Read the model definition and answer for the solid it produces. Units are mm, in the model's axes. A direction names the side the tool comes from. Coordinates: 2 decimals unless noted, no trailing zeros. Loops run counter-clockwise (first coordinate to the right, second up) from the corner with the lowest first, then second, coordinate; pieces in that order, holes last.
Q1. Straight lines are drawn through the part: line 1 (Y direction, x = 22.5, z = 268); line 2 (X direction, y = 24.6, z = 57.15). For each, find the intervals that lie inside material, in ascending order.
Q2. Which of the six approach directions +Z, -Z, +X, -X, +Y, -Y give full straight-line access (tool end or side, diameter ignored) to faces 4 (the face through (13, 0, 244)), 5 (the face through (23.812, 13, 243))?
Q3. The mould has two halves that part along Y. Classify faces 1 (the face through (13, 1.588, 243)), 2 (the face through (1, 13, 0)), 3 (the face through (13, 25.4, 244)): pulls with the +Y half, pulls with the -Y half, needs draft (parallel to the pull), parting line crosses it, or undercut.
Q4. Section A-A (z = 274) is taken. Give the vertices of the cut face in (x, y).
Autodesk Inventor part; units mm, degrees
ref_plane "YZ Plane" through (0, 0, 0) normal (1, 0, 0) x (0, 1, 0)
ref_plane "XZ Plane" through (0, 0, 0) normal (0, 1, 0) x (-1, 0, 0)
ref_plane "XY Plane" through (0, 0, 0) normal (0, 0, 1) x (1, 0, 0)
sketch "Sketch1" plane through (0, 0, 0) normal (0, 0, 1) x (1, 0, 0)
  line L0 (0, 0) -> (25.4, 0)
  line L1 (25.4, 0) -> (25.4, 25.4)
  line L2 (25.4, 25.4) -> (0, 25.4)
  line L3 (0, 25.4) -> (0, 0)
  line L4 (1.5875, 23.8125) -> (23.8125, 23.8125)
  line L5 (23.8125, 23.8125) -> (23.8125, 1.5875)
  line L6 (23.8125, 1.5875) -> (1.5875, 1.5875)
  line L7 (1.5875, 1.5875) -> (1.5875, 23.8125)
  dimension "d0" = 25.4
  dimension "d1" = 25.4
  dimension "d2" = 1.5875
extrude "Extrusion1" add sketch "Sketch1" along normal blind 495.3
sketch "Sketch2" plane through (0, 25.4, 0) normal (0, 1, 0) x (1, 0, 0)
  line L0 (25.4, 0) -> (0, 0)
  line L1 (0, 0) -> (0, -495.3)
  line L2 (25.4, -495.3) -> (0, -495.3)
  line L3 (12.7, 0) -> (12.7, -495.3) construction
  line L4 (25.4, -495.3) -> (0, -469.9)
  circle A0 centre (12.7, -79.375) radius 3.3782
  circle A1 centre (12.7, -57.15) radius 3.3782
  circle A2 centre (12.7, -438.15) radius 3.3782
  circle A3 centre (12.7, -415.925) radius 3.3782
  circle A4 centre (11.9062, -191.2218) radius 3.3782
  circle A5 centre (11.9062, -232.4968) radius 3.3782
  line L5 (-2.6988, -143.5968) -> (-2.6988, -242.0218) construction
  line L6 (24.6062, -242.0218) -> (-2.6988, -242.0218) construction
  line L7 (24.6062, -143.5968) -> (24.6062, -242.0218)
  line L8 (-2.6988, -143.5968) -> (24.6062, -143.5968) construction
  dimension "d6" = 45
extrude "Extrusion2" cut sketch "Sketch2" against normal blind 25.4
sketch "Sketch3" plane through (25.4, 0, 0) normal (1, 0, 0) x (0, 0, -1)
  circle A0 centre (-149.9468, 12.7434) radius 3.3782
  circle A1 centre (-175.3468, 12.7434) radius 3.3782
  circle A2 centre (-406.4, 12.7) radius 3.3782
  circle A3 centre (-457.2, 12.7) radius 3.3782
extrude "Extrusion3" cut sketch "Sketch3" against normal blind 25.4
properties part number "Rebuild Shooter Tower Top Tube 1" material "Aluminum 6061"
Numbers:
1. line 1: y = 0 to 1.59, 23.81 to 25.4
1. line 2: x = 0 to 9.32, 16.08 to 25.4
2. face 4: +Z, -Z, +X, -X, -Y
2. face 5: +Z, -Z
3. face 1: undercut
3. face 2: needs draft
3. face 3: pulls with the +Y half
4. outline: (0, 0) - (25.4, 0) - (25.4, 25.4) - (0, 25.4) - close; hole (1.59, 1.59) - (23.81, 1.59) - (23.81, 23.81) - (1.59, 23.81) - close
